Check sheet for the modelled part. Datum: model origin and axes. Units: mm. A direction names the side the tool comes from. Coordinates: 2 decimals unless noted, no trailing zeros. Loops run counter-clockwise (first coordinate to the right, second up) from the corner with the lowest first, then second, coordinate; pieces in that order, holes last. Notation, with made-up numbers: (-3.75, 49) - (49.25, 49) arc R16 cw to (49.25, 65) - close; hole circle Ø1 at (25.5, 32.25). An arc over 180 degrees is marked (long way). Answer as a JSON object with one key per item and string values. Group by question number.
from build123d import *

# Parameters (mm, degrees)
CROQUIS1_R              = 35
SALIENTE_EXTRUIR1_DEPTH = 15
CROQUIS2_R              = 8
CORTAR_EXTRUIR1_DEPTH   = 52.720402164
VACIADO1_T              = -2
REDONDEO1_R             = 2
REDONDEO2_R             = 4
CORTAR_EXTRUIR2_START   = -25
CORTAR_EXTRUIR2_DEPTH   = 27.720402164


with BuildPart() as part:
    # Croquis1 → Saliente-Extruir1 (new body)
    with BuildSketch(Plane.XY):
        Circle(CROQUIS1_R)
    extrude(amount=SALIENTE_EXTRUIR1_DEPTH)

    # Croquis2 → Cortar-Extruir1 (cut, through all)
    with BuildSketch(Plane.XY.offset(15)):
        Circle(CROQUIS2_R)
    extrude(amount=-CORTAR_EXTRUIR1_DEPTH, mode=Mode.SUBTRACT)

    # Vaciado1
    vaciado1_openings = [part.faces().sort_by_distance(p)[0] for p in [
        (-34.010050506, 0, 15),
    ]]
    offset(amount=VACIADO1_T, openings=vaciado1_openings, kind=Kind.INTERSECTION)

    # Redondeo1
    redondeo1_edges = [part.edges().sort_by_distance(p)[0] for p in [
        (-33, 0, 2),
    ]]
    fillet(redondeo1_edges, radius=REDONDEO1_R)

    # Redondeo2
    redondeo2_edges = [part.edges().sort_by_distance(p)[0] for p in [
        (-35, 0, 0),
    ]]
    fillet(redondeo2_edges, radius=REDONDEO2_R)

    # Croquis3 → Cortar-Extruir2 (cut, through all)
    with BuildSketch(Plane(origin=(0, 0, 0), x_dir=(1, 0, 0), z_dir=(0, 1, 0)).offset(CORTAR_EXTRUIR2_START)):
        with BuildLine():
            Line((-5, -2), (5, -2))
            ThreePointArc((5, -2), (7, -4), (5, -6))
            Line((5, -6), (-5, -6))
            ThreePointArc((-5, -6), (-7, -4), (-5, -2))
        make_face()
    extrude(amount=-CORTAR_EXTRUIR2_DEPTH, mode=Mode.SUBTRACT)


solid = part.part
1. Release check for a two-part mould opening along X. For faces 4 (the face through (-28, -21, 9)), 5 (the face through (0, 8.2, 15)), 6 (the face through (-7, -33, 4)) record: released by +X, released by -X, zero draft, split by the parting line, or undercut.
2. Gauge pin test, flat ends, axial feed: pin 1 (1.5 mm diameter, centred on x = -27, y = 6, fed in from -Z); pin 2 (1.9 mm diameter, centred on x = 0, y = -34, fed in from -Z); pin 3 (1 mm diameter, centred on x = -18.5, z = 6, fed in from +Y); pin 4 (6 mm diameter, centred on x = 27.5, z = 3.5, fed in from -Y). Record the tip position at first contact, or that the pin passes through.
3. Access from +Z, -Z, +X, -X, +Y, -Y to the whole of each face (thin tool, end or side, straight path). Record for faces 1 (the face through (-1.73, -7.81, 7.6)), 2 (the face through (-2.17, -9.76, 8.59)), 3 (the face through (7, -33, 4)).
4. Sectioned sample at A-A on x = 0. Record the cut outline in (y, z), plus the area to 3 significant figures.
5. Sectioned sample at C-C on y = 0. Record the cut outline in (x, z).
6. Material ranges on line 1 (Y direction, x = 0, z = 10); line 2 (X direction, y = 1, z = 4.5); line 3 (Z direction, x = -20, y = -8), recorded low to high.
7. Sectioned sample at B-B on z = 7. Record the cut outline in (x, y).
Answers follow:
{
 "1": {"face 4": "split by the parting line", "face 5": "zero draft", "face 6": "undercut"},
 "2": {"pin 1": "stops at z = 0", "pin 2": "stops at z = 0.57", "pin 3": "stops at y = 30.02", "pin 4": "stops at y = -24.97"},
 "3": {"face 1": "+Z, -Z", "face 2": "+Z", "face 3": "-Y"},
 "4": {"outline": "(-35, 6) - (-33, 6) - (-33, 15) - (-35, 15) - close; (-34.46, 2) arc R4 ccw to (-31, 0) - (-8, 0) - (-8, 15) - (-10, 15) - (-10, 2) - close; (8, 0) - (31, 0) arc R4 ccw to (35, 4) - (35, 15) - (33, 15) - (33, 4) arc R2 cw to (31, 2) - (10, 2) - (10, 15) - (8, 15) - close", "area": "198 mm^2"},
 "5": {"outline": "(-35, 4) arc R4 ccw to (-31, 0) - (-8, 0) - (-8, 15) - (-10, 15) - (-10, 2) - (-31, 2) arc R2 cw to (-33, 4) - (-33, 15) - (-35, 15) - close; (8, 0) - (31, 0) arc R4 ccw to (35, 4) - (35, 15) - (33, 15) - (33, 4) arc R2 cw to (31, 2) - (10, 2) - (10, 15) - (8, 15) - close"},
 "6": {"line 1": "y = -35 to -33, -10 to -8, 8 to 10, 33 to 35", "line 2": "x = -34.99 to -32.98, -9.95 to -7.94, 7.94 to 9.95, 32.98 to 34.99", "line 3": "z = 0 to 2"},
 "7": {"outline": "circle Ø70 at (0, 0); circle Ø20 at (0, 0); hole circle Ø66 at (0, 0); hole circle Ø16 at (0, 0)"}
}
